Job drawing, mm, ordinate dimensions from the low corner. One solid piece. Round coordinates to 2 decimals unless told otherwise and drop trailing zeros. Write each loop counter-clockwise with the first axis right and the second up, starting at its lowest first coordinate (ties: lowest second). Pieces come first, ordered by that corner, then holes.
1) Saw through at B-B on y = 0.5. Count the separate pieces of the cut face and the enclosed holes in it, and give its area (3 significant figures).
2) Flat gauge pin, fed straight in: pin 1 (0.9 mm diameter, centred on x = 8.89, z = 17.78, fed in from -Y). Where does the tip first touch, or does it go through?
3) Saw through at A-A on x = 11.43. Write the cut outline in (y, z).
4) Drill centre lines: L1, parallel to X at y = 0.8, z = 2.5; L2, parallel to Z at x = 13.97, y = 0.9; L3, parallel to X at y = 1.45, z = 3. Where is each one in solid material? Low to high.
5) Saw through at C-C on x = 16.75. Write the cut outline in (y, z), and give its area (3 significant figures).
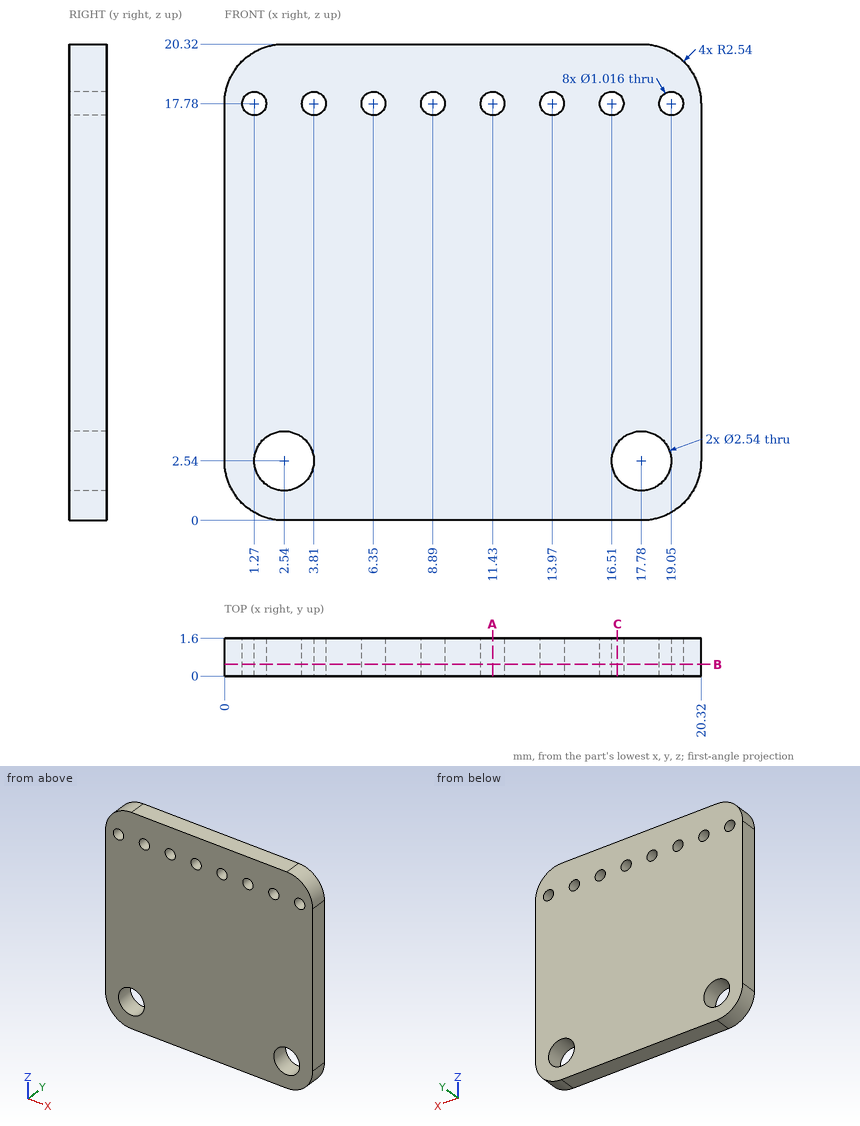
Completed:
1. separate pieces: 1
1. enclosed holes: 10
1. area: 391 mm2
2. pin 1: passes through
3. outline: (0, 0) - (1.6, 0) - (1.6, 17.27) - (0, 17.27) - close; (0, 18.29) - (1.6, 18.29) - (1.6, 20.32) - (0, 20.32) - close
4. L1: x = 0 to 1.27, 3.81 to 16.51, 19.05 to 20.32
4. L2: z = 0 to 17.27, 18.29 to 20.32
4. L3: x = 0 to 1.36, 3.72 to 16.6, 18.96 to 20.32
5. outline: (0, 0) - (1.6, 0) - (1.6, 1.8) - (0, 1.8) - close; (0, 3.28) - (1.6, 3.28) - (1.6, 17.33) - (0, 17.33) - close; (0, 18.23) - (1.6, 18.23) - (1.6, 20.32) - (0, 20.32) - close
5. area: 28.7 mm2
